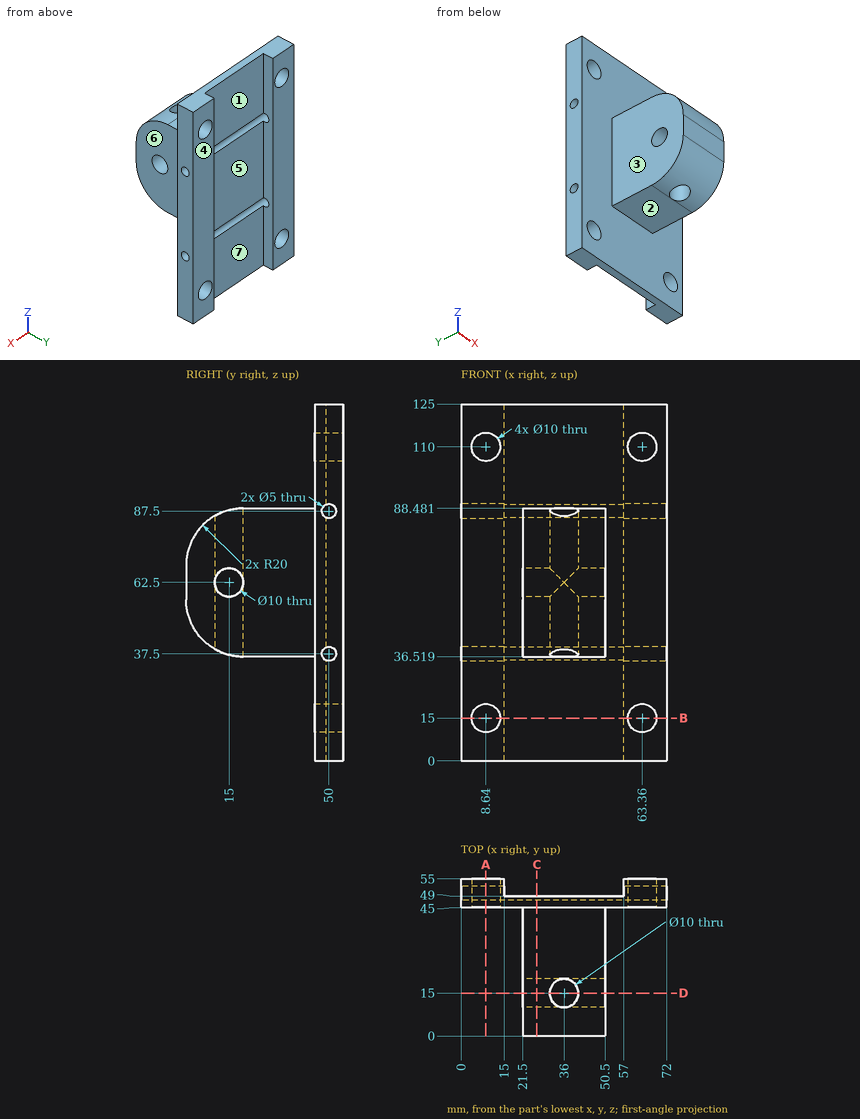
Here's the drawing with two shaded views (mm, measured from the low corner). I have some questions. A direction names the side the tool comes from. Give positions to 0.01 mm unless a question says otherwise; leave off trailing zeros. Loops run counter-clockwise (first coordinate to the right, second up) from the corner with the lowest first, then second, coordinate; pieces in that order, holes last. Notation, with made-up numbers: M 41.25,-31 L 74.25,-31 A28 cw 74.25,4 Z; hole C -38.75,76.5 d10. An arc over 180 degrees is marked long. Answer in a Markdown table with one row per item.
1. Suppose I cut it at D-D on y = 15. Write out the boundary of the cut face in (x, z).
Taken from the geometry:
| item | result |
|---|---|
| outline | M 21.5,37.15 L 31,37.15 L 31,57.5 L 21.5,57.5 Z; M 21.5,67.5 L 31,67.5 L 31,87.85 L 21.5,87.85 Z; M 41,37.15 L 50.5,37.15 L 50.5,57.5 L 41,57.5 Z; M 41,67.5 L 50.5,67.5 L 50.5,87.85 L 41,87.85 Z |
2. Suppose I cut it at A-A on x = 8.64. Write out the boundary of the cut face in (y, z).
Taken from the geometry:
| item | result |
|---|---|
| outline | M 45,0 L 55,0 L 55,10 L 45,10 Z; M 45,20 L 55,20 L 55,105 L 45,105 Z; M 45,115 L 55,115 L 55,125 L 45,125 Z; hole C 50,37.5 d5; hole C 50,87.5 d5 |
3. For pin 1 Ø13 at (x, z) = (63.36, 15) entering from -Y; pin 2 Ø11.5 at (x, z) = (63.36, 110) entering from +Y; pin 3 Ø11.5 at (y, z) = (15, 62.5) entering from +X; pin 4 Ø6 at (x, y) = (36, 15) entering from -Z, each with a flat end and sliding along its axis, tell me the tip position at first contact or that it passes through.
Taken from the geometry:
| item | result |
|---|---|
| pin 1 | stops at y = 45 |
| pin 2 | stops at y = 55 |
| pin 3 | stops at x = 50.5 |
| pin 4 | passes through |
4. If I drill on line 1 along Y through (x, z) = (47, 62) (1 decimal); line 2 along X through (y, z) = (47.25, 110); line 3 along X through (y, z) = (51.5, 28.5), over which ranges is the centre line in solid material (lowest first)?
Taken from the geometry:
| item | result |
|---|---|
| line 1 | y = 0 to 10, 20 to 49 |
| line 2 | x = 0 to 3.64, 13.64 to 58.36, 68.36 to 72 |
| line 3 | x = 0 to 15, 57 to 72 |
5. Suppose I cut it at B-B on z = 15. Write out the boundary of the cut face in (x, y), plus the area to 3 significant figures.
Taken from the geometry:
| item | result |
|---|---|
| outline | M 0,45 L 3.64,45 L 3.64,55 L 0,55 Z; M 13.64,45 L 58.36,45 L 58.36,55 L 57,55 L 57,49 L 15,49 L 15,55 L 13.64,55 Z; M 68.36,45 L 72,45 L 72,55 L 68.36,55 Z |
| area | 268 mm² |
6. Which directions (+Z, -Z, +X, -X, +Y, -Y) give clear straight access to the entire face, cutting with the end or side of a thin tool? Please do the marked faces 1, 2 and 3.
Taken from the geometry:
| item | result |
|---|---|
| face 1 | +Z, -Z, +Y |
| face 2 | -Z, +X, -X, -Y |
| face 3 | +Z, -Z, -X, -Y |
7. Thinking about a two-plate mould opening in X: for the marked faces 4, 5, 6 and 7, which applies, released by +X, released by -X, zero draft, split by the parting line, or undercut?
Taken from the geometry:
| item | result |
|---|---|
| face 4 | zero draft |
| face 5 | undercut |
| face 6 | released by +X |
| face 7 | undercut |
8. Suppose I cut it at C-C on x = 26.5. Write out the boundary of the cut face in (y, z).
Taken from the geometry:
| item | result |
|---|---|
| outline | M 0,56.52 A20 ccw 20,36.52 L 45,36.52 L 45,0 L 49,0 L 49,35.21 A2.5 cw 49,39.79 L 49,85.21 A2.5 cw 49,89.79 L 49,125 L 45,125 L 45,88.48 L 20,88.48 A20 ccw 0,68.48 Z; hole C 15,62.5 d10 |
